```python
from build123d import *

# Parameters (mm, degrees)
F0_W     = 30
F0_H     = 15
F1_DEPTH = 14
F3_R     = 2.5
F4_DEPTH = 14.001
F5_R     = 5
F6_DEPTH = 14.001
F7_W     = 55
F7_H     = 17
F8_DEPTH = 14.001
F2_R     = 5.5
F9_DEPTH = 85.001


with BuildPart() as f1:
    # F0 (on Top) → F1 (new body)
    with BuildSketch(Plane.XY):
        Polygon((27.5, 25), (-27.5, 25), (-27.5, -25), (27.5, -25), (27.5, -10), align=None)
        with Locations((42.5, -17.5)):
            Rectangle(F0_W, F0_H)
    extrude(amount=F1_DEPTH)

    # F3 (on face) → F4 (cut, through all)
    with BuildSketch(Plane.XY.offset(14)):
        with Locations((0, -15)):
            Circle(F3_R)
    extrude(amount=-F4_DEPTH, mode=Mode.SUBTRACT)

    # F5 (on face) → F6 (cut, through all)
    with BuildSketch(Plane.XY.offset(14)):
        with Locations((49.511172, -17.922652)):
            Circle(F5_R)
    extrude(amount=-F6_DEPTH, mode=Mode.SUBTRACT)

    # F7 (on face) → F8 (cut, through all)
    with BuildSketch(Plane(origin=(0, 0, 0), x_dir=(1, 0, 0), z_dir=(0, 0, -1))):
        with Locations((0, -16.5)):
            Rectangle(F7_W, F7_H)
    extrude(amount=-F8_DEPTH, mode=Mode.SUBTRACT)

    # F2 (on face) → F9 (cut, through all)
    with BuildSketch(Plane(origin=(-27.5, 0, 0), x_dir=(0, -1, 0), z_dir=(-1, 0, 0))):
        with Locations((0, 6.5)):
            Circle(F2_R)
    extrude(amount=-F9_DEPTH, mode=Mode.SUBTRACT)


solid = f1.part
```
The model under review builds one solid part; all positions refer to its coordinate system, in mm. A direction names the side the tool comes from. Round coordinates to 2 decimals unless told otherwise and drop trailing zeros. Order: outer loops, then holes, each group sorted by start corner. A loop starts at its lowest first (then second) coordinate and runs counter-clockwise, first axis right, second up.
Item 1: Add section C-C, the plane x = 3.5. State the section outline as (y, z) points.
Working result:
outline: (-25, 0) - (8, 0) - (8, 14) - (-25, 14) - close; hole circle Ø11 at (0, 6.5)
Item 2: To check wall thickness, follow probe 1 along Z at (x, y) = (-10, 0); probe 2 along Y at (x, z) = (34, 13); probe 3 along Y at (x, z) = (1, 8.25). State the ranges of each line that lie inside material, in increasing order.
Working result:
probe 1: z = 0 to 1, 12 to 14
probe 2: y = -25 to -10
probe 3: y = -25 to -17.29, -12.71 to -5.21, 5.21 to 8
Item 3: Add section B-B, the plane z = 8. State the section outline as (x, y) points, and give its area (3 significant figures).
Working result:
outline: (-27.5, -25) - (57.5, -25) - (57.5, -10) - (27.5, -10) - (27.5, -5.29) - (-27.5, -5.29) - close; (-27.5, 5.29) - (27.5, 5.29) - (27.5, 8) - (-27.5, 8) - close; hole circle Ø5 at (0, -15); hole circle Ø10 at (49.51, -17.92)
area: 1,580 mm2
Item 4: Machinability: for faces 4 (the flat face through (42, -10, 7)), 5 (the flat face through (14, -25, 7)), which of the approach directions +Z, -Z, +X, -X, +Y, -Y give a long, thin tool a straight path to every point of the face, cutting with its end or side? Answer none if there is none.
Working result:
face 4: +Z, -Z, +X, +Y
face 5: +Z, -Z, +X, -X, -Y
Item 5: Draft analysis for pull direction Y (two halves, no side actions). For faces 1 (the cylindrical face through (-0.54, -17.44, 7.1)), 2 (the flat face through (5, -8, 0)), 3 (the flat face through (0, 8, 7)), state which applies: released by +Y, released by -Y, zero draft, split by the parting line, or undercut.
Working result:
face 1: undercut
face 2: zero draft
face 3: released by +Y
Item 6: Add section D-D, the plane z = 3. State the section outline as (x, y) points, and give its area (3 significant figures).
Working result:
outline: (-27.5, -25) - (57.5, -25) - (57.5, -10) - (27.5, -10) - (27.5, -4.24) - (-27.5, -4.24) - close; (-27.5, 4.24) - (27.5, 4.24) - (27.5, 8) - (-27.5, 8) - close; hole circle Ø5 at (0, -15); hole circle Ø10 at (49.51, -17.92)
area: 1,700 mm2
Item 7: Add section A-A, the plane y = 0. State the section outline as (x, z) points.
Working result:
outline: (-27.5, 0) - (27.5, 0) - (27.5, 1) - (-27.5, 1) - close; (-27.5, 12) - (27.5, 12) - (27.5, 14) - (-27.5, 14) - close
